Part model, mm, in its own coordinate system. Give positions to 0.01 mm unless a question says otherwise; leave off trailing zeros. Order: outer loops, then holes, each group sorted by start corner. A loop starts at its lowest first (then second) coordinate and runs counter-clockwise, first axis right, second up. Notation, with made-up numbers: (88, -6.75) -> (107, -6.75) arc R18 ccw to (107, 27.25) -> close; hole circle Ø1 at (60, 67.5). An arc over 180 degrees is marked (long way). Write item = value, one per line. Start each with the question number.
(1) Saw through at C-C, the plane x = -2.5. List the corners of the cut face in (y, z), then the cut area to 3 significant figures.
(2) Saw through at B-B, the plane z = 31. List the corners of the cut face in (x, y), then the cut area to 3 significant figures.
(3) Saw through at A-A, the plane y = -13.5. List the corners of the cut face in (x, z) (3 decimals), then the cut area to 3 significant figures.
(4) Probe line 1 along Z through (x, y) = (-4, -7.75); line 2 along Z through (x, y) = (96.5, -4.25); line 3 along Z through (x, y) = (-105.5, -14). List the from-to ranges inside material, lowest first. Write a range as from..to.
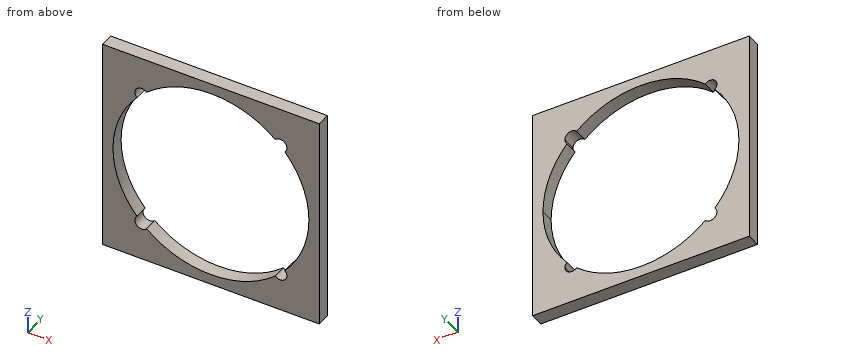
from build123d import *

# Parameters (mm, degrees)
F0_W     = 304.8
F0_H     = 304.8
F1_DEPTH = 19.05


with BuildPart() as f1:
    # F0 (on Front) → F1 (new body)
    with BuildSketch(Plane.XZ):
        Rectangle(F0_W, F0_H)
        with BuildLine():
            ThreePointArc((103.934164, 90.471828), (129.052451, 48.300383), (137.795, 0))
            ThreePointArc((137.795, 0), (129.052451, -48.300383), (103.934164, -90.471828))
            ThreePointArc((103.934164, -90.471828), (106.171417, -93.639168), (106.960779, -97.435779))
            ThreePointArc((106.960779, -97.435779), (100.928198, -106.297417), (90.471828, -103.934164))
            ThreePointArc((90.471828, -103.934164), (0, -137.795), (-90.471828, -103.934164))
            ThreePointArc((-90.471828, -103.934164), (-104.170971, -104.170971), (-103.934164, -90.471828))
            ThreePointArc((-103.934164, -90.471828), (-137.795, 0), (-103.934164, 90.471828))
            ThreePointArc((-103.934164, 90.471828), (-104.170971, 104.170971), (-90.471828, 103.934164))
            ThreePointArc((-90.471828, 103.934164), (0, 137.795), (90.471828, 103.934164))
            ThreePointArc((90.471828, 103.934164), (100.928198, 106.297417), (106.960779, 97.435779))
            ThreePointArc((106.960779, 97.435779), (106.171417, 93.639168), (103.934164, 90.471828))
        make_face(mode=Mode.SUBTRACT)
    extrude(amount=F1_DEPTH)


solid = f1.part
Results list:
q1.outline = (-19.05, -152.4) -> (0, -152.4) -> (0, -137.77) -> (-19.05, -137.77) -> close; (-19.05, 137.77) -> (0, 137.77) -> (0, 152.4) -> (-19.05, 152.4) -> close
q1.area = 557 mm^2
q2.outline = (-152.4, -19.05) -> (-134.26, -19.05) -> (-134.26, 0) -> (-152.4, 0) -> close; (134.26, -19.05) -> (152.4, -19.05) -> (152.4, 0) -> (134.26, 0) -> close
q2.area = 691 mm^2
q3.outline = (-152.4, -152.4) -> (152.4, -152.4) -> (152.4, 152.4) -> (-152.4, 152.4) -> close; hole (-103.934, -90.472) arc R9.525 ccw (long way) to (-90.472, -103.934) arc R137.795 ccw to (90.472, -103.934) arc R9.525 ccw to (106.961, -97.436) arc R9.525 ccw to (103.934, -90.472) arc R137.795 ccw to (137.795, 0) arc R137.795 ccw to (103.934, 90.472) arc R9.525 ccw to (106.961, 97.436) arc R9.525 ccw to (90.472, 103.934) arc R137.795 ccw to (-90.472, 103.934) arc R9.525 ccw (long way) to (-103.934, 90.472) arc R137.795 ccw to start
q3.area = 32,700 mm^2
q4.line_1 = -152.4..-137.74, 137.74..152.4
q4.line_2 = -152.4..-106.91, 106.91..152.4
q4.line_3 = -152.4..-102.5, -92.37..-88.64, 88.64..92.37, 102.5..152.4
